Build history of the part. All positions in model axes, mm. A direction names the side the tool comes from. Give positions to 0.01 mm unless a question says otherwise; leave off trailing zeros. Loops run counter-clockwise (first coordinate to the right, second up) from the corner with the lowest first, then second, coordinate; pieces in that order, holes last. Notation, with made-up numbers: M 38,83.5 L 87,83.5 A25 ccw 87,117.5 Z; hole C 19,36.25 d11. An arc over 180 degrees is marked long. Answer as a JSON object with one key per item and string values. Group by question number.
1. Slice it at C-C (z = 21.75). List the corners of the cut face in (x, y), then the cut area to 3 significant figures.
2. Mould opens along Z. For faces 4 (the face through (1, -2.339, 13)), 5 (the face through (0, -6, 18)), 6 (the face through (0.8, -9.6, 12.8)), 7 (the face through (1, -2, 9.573)) say: released by +Z, released by -Z, zero draft, split by the parting line, or undercut.
3. 3-axis set-ups, long thin cutter, end or side, ignore diameter. For faces 1 (the face through (0.783, -1.047, 20.018)), 2 (the face through (1, -2, 15.923)), 3 (the face through (0.783, -2.1, 20.666)): which of +Z, -Z, +X, -X, +Y, -Y reach the whole face in a straight line?
4. Slice it at B-B (y = -4.25). List the corners of the cut face in (x, z).
5. Slice it at A-A (x = 0.9). List the corners of the cut face in (y, z).
6. Drill centre lines: line 1 along Y through (x, z) = (1.35, 13.25); line 2 along Y through (x, z) = (0.9, 22.5); line 3 along Z through (x, y) = (0.7, -10.25). Where is each one in solid material? Low to high. Write a range as [from, to].
7. Drop a flat-ended pin along its axis: pin 1 Ø0.5 at (x, y) = (1, -1.5) entering from +Z. Give the stop position or say it passes through.
8. Slice it at D-D (y = -1.75). List the corners of the cut face in (x, z).
from build123d import *

# Parameters (mm, degrees)
BOSS_EXTRUDE1_DEPTH = 1.5875


with BuildPart() as part:
    # Sketch1 → Boss-Extrude1 (new body)
    with BuildSketch(Plane(origin=(0, 0, 0), x_dir=(0, 0, -1), z_dir=(1, 0, 0))):
        with BuildLine():
            Line((-6.398003714, -0.75184), (-6.398003714, -2.33934))
            Line((-6.398003714, -2.33934), (-19.419469424, -17.102153274))
            ThreePointArc((-19.419469424, -17.102153274), (-25.055238608, -7.661312267), (-35.94689414, -6.156914384))
            Line((-35.94689414, -6.156914384), (-26.958444364, -3.273446191))
            Line((-26.958444364, -3.273446191), (-26.473520097, -4.785069393))
            Line((-26.473520097, -4.785069393), (-20.427027289, -2.845372323))
            Line((-20.427027289, -2.845372323), (-20.911951556, -1.333749121))
            Line((-20.911951556, -1.333749121), (-19.098003714, -0.75184))
            Line((-19.098003714, -0.75184), (-15.923003714, -0.75184))
            Line((-15.923003714, -0.75184), (-15.923003714, -2.33934))
            Line((-15.923003714, -2.33934), (-9.573003714, -2.33934))
            Line((-9.573003714, -2.33934), (-9.573003714, -0.75184))
            Line((-9.573003714, -0.75184), (-6.398003714, -0.75184))
        make_face()
    extrude(amount=BOSS_EXTRUDE1_DEPTH)


solid = part.part
Established:
{
 "1": {"outline": "M 0,-10.84 L 1.59,-10.84 L 1.59,-3.27 L 0,-3.27 Z", "area": "12.0 mm^2"},
 "2": {"face 4": "undercut", "face 5": "zero draft", "face 6": "released by -Z", "face 7": "undercut"},
 "3": {"face 1": "+Z, +X, -X, +Y", "face 2": "+X, -X, +Y", "face 3": "+Z, +X, -X"},
 "4": {"outline": "M 0,8.08 L 1.59,8.08 L 1.59,24.81 L 0,24.81 Z; M 0,26.65 L 1.59,26.65 L 1.59,30 L 0,30 Z"},
 "5": {"outline": "M -17.1,19.42 L -2.34,6.4 L -0.75,6.4 L -0.75,9.57 L -2.34,9.57 L -2.34,15.92 L -0.75,15.92 L -0.75,19.1 L -1.33,20.91 L -2.85,20.43 L -4.79,26.47 L -3.27,26.96 L -6.16,35.95 A12.7 cw Z"},
 "6": {"line 1": "y = [-10.11, -2.34]", "line 2": "y = [-9.9, -3.51]", "line 3": "z = [13.38, 22.2]"},
 "7": {"pin 1": "stops at z = 20.91"},
 "8": {"outline": "M 0,6.4 L 1.59,6.4 L 1.59,9.57 L 0,9.57 Z; M 0,15.92 L 1.59,15.92 L 1.59,20.78 L 0,20.78 Z"}
}
